from build123d import *

# Parameters (mm, degrees)
F0_R      = 50
F1_DEPTH  = 5
F2_R      = 6
F3_DEPTH  = 1
F4_R      = 4.3
F5_DEPTH  = 7
F7_D      = 2.65
F7_DEPTH  = 5
F7_TIP    = 0.7961403202
F8_SIZE2  = 2
F8_SIZE   = 0.2
F9_R      = 4
F10_DEPTH = 1


# Not quite as in the source:
# - a fillet or chamfer that OpenCascade refuses, or shapes differently, is made with other operations: its cross-section is extruded or revolved along the edge and cut away or added


with BuildPart() as f1:
    # F0 (on Top) → F1 (new body)
    with BuildSketch(Plane.XY):
        Circle(F0_R)
    extrude(amount=F1_DEPTH)

    # F2 (on face) → F3 (join)
    with BuildSketch(Plane.XY.offset(5)):
        Circle(F2_R)
    extrude(amount=F3_DEPTH)

    # F4 (on face) → F5 (join)
    with BuildSketch(Plane.XY.offset(6)):
        Circle(F4_R)
    extrude(amount=F5_DEPTH)

    # F7
    with Locations(Plane.XY.offset(13)):
        with Locations((0, 0)):
            Hole(F7_D / 2, depth=F7_DEPTH)
            with Locations((0, 0, -(F7_DEPTH + F7_TIP / 2))):  # 118° drill point
                Cone(0, F7_D / 2, F7_TIP, mode=Mode.SUBTRACT)

    # F8
    f8_edges = [f1.edges().sort_by_distance(p)[0] for p in [
        (-4.3, 0, 13),
    ]]
    f8_side = f1.faces().sort_by_distance((-4.178378, 0, 13))[0]
    chamfer(f8_edges, length=F8_SIZE, length2=F8_SIZE2, reference=f8_side)

    # F9 (on face) → F10 (join)
    with BuildSketch(Plane.XY.offset(5)):
        with Locations((0, 45)):
            Circle(F9_R)
        with Locations((-31.8198051534, 31.8198051534)):
            Circle(F9_R)
        with Locations((-45, 0)):
            Circle(F9_R)
        with Locations((-31.8198051534, -31.8198051534)):
            Circle(F9_R)
        with Locations((0, -45)):
            Circle(F9_R)
        with Locations((31.8198051534, -31.8198051534)):
            Circle(F9_R)
        with Locations((45, 0)):
            Circle(F9_R)
        with Locations((31.8198051534, 31.8198051534)):
            Circle(F9_R)
    extrude(amount=F10_DEPTH)

    # F11: fillet of radius 5 on 8 edges, made by hand

    # F11_s1 → F11_t2 (revolve, cut)
    with BuildSketch(Plane.XZ.offset(45)):
        with BuildLine():
            ThreePointArc((4, 5), (2.5811388301, 5.7434164903), (1, 6))
            Line((1, 6), (4, 6))
            Line((4, 6), (4, 5))
        make_face()
    revolve(axis=Axis((0, -45, 6), (0, 0, 1)), mode=Mode.SUBTRACT)

    # F11_s3 → F11_t4 (revolve, cut)
    with BuildSketch(Plane.XZ.offset(31.8198051534)):
        with BuildLine():
            ThreePointArc((35.8198051534, 5), (34.4009439835, 5.7434164903), (32.8198051534, 6))
            Line((32.8198051534, 6), (35.8198051534, 6))
            Line((35.8198051534, 6), (35.8198051534, 5))
        make_face()
    revolve(axis=Axis((31.8198051534, -31.8198051534, 6), (0, 0, 1)), mode=Mode.SUBTRACT)

    # F11_s5 → F11_t6 (revolve, cut)
    with BuildSketch(Plane.XZ):
        with BuildLine():
            ThreePointArc((49, 5), (47.5811388301, 5.7434164903), (46, 6))
            Line((46, 6), (49, 6))
            Line((49, 6), (49, 5))
        make_face()
    revolve(axis=Axis((45, 0, 6), (0, 0, 1)), mode=Mode.SUBTRACT)

    # F11_s7 → F11_t8 (revolve, cut)
    with BuildSketch(Plane.XZ.offset(-31.8198051534)):
        with BuildLine():
            ThreePointArc((35.8198051534, 5), (34.4009439835, 5.7434164903), (32.8198051534, 6))
            Line((32.8198051534, 6), (35.8198051534, 6))
            Line((35.8198051534, 6), (35.8198051534, 5))
        make_face()
    revolve(axis=Axis((31.8198051534, 31.8198051534, 6), (0, 0, 1)), mode=Mode.SUBTRACT)

    # F11_s9 → F11_t10 (revolve, cut)
    with BuildSketch(Plane.XZ.offset(-45)):
        with BuildLine():
            ThreePointArc((4, 5), (2.5811388301, 5.7434164903), (1, 6))
            Line((1, 6), (4, 6))
            Line((4, 6), (4, 5))
        make_face()
    revolve(axis=Axis((0, 45, 6), (0, 0, 1)), mode=Mode.SUBTRACT)

    # F11_s11 → F11_t12 (revolve, cut)
    with BuildSketch(Plane.XZ.offset(-31.8198051534)):
        with BuildLine():
            ThreePointArc((-27.8198051534, 5), (-29.2386663233, 5.7434164903), (-30.8198051534, 6))
            Line((-30.8198051534, 6), (-27.8198051534, 6))
            Line((-27.8198051534, 6), (-27.8198051534, 5))
        make_face()
    revolve(axis=Axis((-31.8198051534, 31.8198051534, 6), (0, 0, 1)), mode=Mode.SUBTRACT)

    # F11_s13 → F11_t14 (revolve, cut)
    with BuildSketch(Plane.XZ):
        with BuildLine():
            ThreePointArc((-41, 5), (-42.4188611699, 5.7434164903), (-44, 6))
            Line((-44, 6), (-41, 6))
            Line((-41, 6), (-41, 5))
        make_face()
    revolve(axis=Axis((-45, 0, 6), (0, 0, 1)), mode=Mode.SUBTRACT)

    # F11_s15 → F11_t16 (revolve, cut)
    with BuildSketch(Plane.XZ.offset(31.8198051534)):
        with BuildLine():
            ThreePointArc((-27.8198051534, 5), (-29.2386663233, 5.7434164903), (-30.8198051534, 6))
            Line((-30.8198051534, 6), (-27.8198051534, 6))
            Line((-27.8198051534, 6), (-27.8198051534, 5))
        make_face()
    revolve(axis=Axis((-31.8198051534, -31.8198051534, 6), (0, 0, 1)), mode=Mode.SUBTRACT)


solid = f1.part
Geometry: final body of the model. Coordinates: model frame, mm. A direction names the side the tool comes from. Give positions to 0.01 mm unless a question says otherwise; leave off trailing zeros. Write each loop counter-clockwise with the first axis right and the second up, starting at its lowest first coordinate (ties: lowest second). Pieces come first, ordered by that corner, then holes. Notation, with made-up numbers: M 57.25,-17.5 L 103.25,-17.5 A28 cw 103.25,6.5 Z; hole C 34,35 d7. An arc over 180 degrees is marked long. Answer in a Markdown table with one row per item. Add a question column.
(1) Reachability of faces 1 (the flat face through (2, 0, 13)), 2 (the cylindrical face through (-5.994, 0.264, 5.493)) from +Z, -Z, +X, -X, +Y, -Y: full face, straight path, thin tool, end or side. Return the list, or none.
(2) Section C-C on y = 38.5. Return loops of the section in (x, z).
(3) Section B-B on x = 38. Return loops of the section in (y, z), and give its area (3 significant figures).
(4) First-contact query: pin 1 (0.6 mm diameter, centred on x = -31.5, y = -32, fed in from +Z); pin 2 (4 mm diameter, centred on x = -35, y = 37.5, fed in from +Z); pin 3 (5 mm diameter, centred on y = -2.5, z = 10, fed in from +X); pin 4 (2 mm diameter, centred on x = 0, y = 0, fed in from -Z). Flat tips, straight axial feed; report the tip coordinate or a pass-through.
(5) Mould query, pull axis Y, two halves, no side actions, for faces 3 (the flat face through (3, -4, 6)), 4 (the cylindrical face through (-1.224, -0.507, 10.465)), 5 (the cylindrical face through (-4.296, 0.189, 8.465)). Classes: +Y half, -Y half, draft (parallel to the pull), parting line (faces both ways), or undercut.
(6) Ray query, line 1 (Y direction, x = 0, z = 10.2) (3 decimals); line 2 (Z direction, x = -22, y = 21.5); line 3 (Y direction, x = 0, z = 11.5) (3 decimals). Return the intervals inside material, ascending.
(7) Section A-A on z = 3.25. Return loops of the section in (x, y).
Result set:
| question | item | result |
|---|---|---|
| 1 | face 1 | +Z, +X, -X, +Y, -Y |
| 1 | face 2 | +Z |
| 2 | outline | M -31.9,0 L 31.9,0 L 31.9,5 L -31.9,5 Z |
| 3 | outline | M -32.5,0 L 32.5,0 L 32.5,5 L -32.5,5 Z |
| 3 | area | 325 mm^2 |
| 4 | pin 1 | stops at z = 6 |
| 4 | pin 2 | stops at z = 5 |
| 4 | pin 3 | stops at x = 4.3 |
| 4 | pin 4 | stops at z = 0 |
| 5 | face 3 | draft |
| 5 | face 4 | undercut |
| 5 | face 5 | parting line |
| 6 | line 1 | y = -4.3 to -1.325, 1.325 to 4.3 |
| 6 | line 2 | z = 0 to 5 |
| 6 | line 3 | y = -4.25 to -1.325, 1.325 to 4.25 |
| 7 | outline | C 0,0 d100 |
